Here's how the part is built. I have some questions about the finished solid (model axes, mm). A direction names the side the tool comes from. Give positions to 0.01 mm unless a question says otherwise; leave off trailing zeros. Order: outer loops, then holes, each group sorted by start corner. A loop starts at its lowest first (then second) coordinate and runs counter-clockwise, first axis right, second up.
from build123d import *

# Parameters (mm, degrees)
F0_R     = 10
F0_R_2   = 7.5
F1_DEPTH = 30
F2_R     = 4
F3_DEPTH = 2.5
F4_R     = 7.5
F5_DEPTH = 30.001


with BuildPart() as f1:
    # F0 (on Front) → F1 (new body)
    with BuildSketch(Plane.XZ):
        Circle(F0_R)
        Circle(F0_R_2, mode=Mode.SUBTRACT)
    extrude(amount=F1_DEPTH)

    # F2 (on Right) → F3 (join, symmetric)
    with BuildSketch(Plane.YZ):
        with BuildLine():
            Line((-22.5, 0.945997), (-7.5, 0.945997))
            Line((-7.5, 0.945997), (-7.5, 30.945997))
            ThreePointArc((-7.5, 30.945997), (-15, 38.445997), (-22.5, 30.945997))
            Line((-22.5, 30.945997), (-22.5, 0.945997))
        make_face()
        with Locations((-15, 30.945997)):
            Circle(F2_R, mode=Mode.SUBTRACT)
        with BuildLine():
            Line((-7.5, -29.054003), (-7.5, 0.945997))
            Line((-7.5, 0.945997), (-22.5, 0.945997))
            Line((-22.5, 0.945997), (-22.5, -29.054003))
            ThreePointArc((-22.5, -29.054003), (-15, -36.554003), (-7.5, -29.054003))
        make_face()
        with Locations((-15, -29.054003)):
            Circle(F2_R, mode=Mode.SUBTRACT)
    extrude(amount=F3_DEPTH, both=True)

    # F4 (on face) → F5 (cut, through all)
    with BuildSketch(Plane.XZ.offset(30)):
        Circle(F4_R)
    extrude(amount=-F5_DEPTH, mode=Mode.SUBTRACT)


solid = f1.part
Q1. If we section it at A-A on y = -15: List the corners of the cut face in (x, z) for me, plus the area to 3 significant figures.
Filled sheet:
outline: (-2.5, -36.55) - (2.5, -36.55) - (2.5, -33.05) - (-2.5, -33.05) - close; (-2.5, -25.05) - (2.5, -25.05) - (2.5, -9.68) arc R10 ccw to (2.5, 9.68) - (2.5, 26.95) - (-2.5, 26.95) - (-2.5, 9.68) arc R10 ccw to (-2.5, -9.68) - close; (-2.5, 34.95) - (2.5, 34.95) - (2.5, 38.45) - (-2.5, 38.45) - close; hole circle Ø15 at (0, 0)
area: 333 mm2
Q2. I need wall thicknesses on L1, parallel to Z at x = 0.5, y = -15; L2, parallel to X at y = -19, z = -12.5; L3, parallel to X at y = -28, z = 3. Which ranges of each line are inside material? Lowest first, please.
Filled sheet:
L1: z = -36.55 to -33.05, -25.05 to -7.48, 7.48 to 26.95, 34.95 to 38.45
L2: x = -2.5 to 2.5
L3: x = -9.54 to -6.87, 6.87 to 9.54
Q3. For faces 4 (the face through (-2.5, -15, 21)), 5 (the face through (4, -30, 7)), 6 (the face through (4, 0, 7)), 7 (the face through (-2.5, -15, -20)), 8 (the face through (2.5, -15, -20)), which set-ups out of +Z, -Z, +X, -X, +Y, -Y let a thin tool reach every point of the face, with its end or its side?
Filled sheet:
face 4: +Z, -X, +Y, -Y
face 5: +Z, -Z, +X, -X, -Y
face 6: +Z, -Z, +X, -X, +Y
face 7: -Z, -X, +Y, -Y
face 8: -Z, +X, +Y, -Y
Q4. I'm going to push flat-ended pins straight in: P1, Ø7.5, axis at y = -12.5, z = 30.5, coming from the -X side; P2, Ø5.5, axis at x = -1, z = 20.5, coming from the -Y side; P3, Ø4, axis at x = -0.5, z = -20.5, coming from the +Y side; P4, Ø6.5, axis at y = -15, z = 30.95, coming from the +X side. Where does each tip first touch, or does it pass through?
Filled sheet:
P1: stops at x = -2.5
P2: stops at y = -22.5
P3: stops at y = -7.5
P4: passes through
Q5. If we section it at D-D on x = -4.75: List the corners of the cut face in (y, z) for me, plus the area to 3 significant figures.
Filled sheet:
outline: (-30, -8.8) - (0, -8.8) - (0, -5.8) - (-30, -5.8) - close; (-30, 5.8) - (0, 5.8) - (0, 8.8) - (-30, 8.8) - close
area: 180 mm2
Q6. If we section it at C-C on x = -1.25: List the corners of the cut face in (y, z) for me.
Filled sheet:
outline: (-30, -9.92) - (-22.5, -9.92) - (-22.5, -29.05) arc R7.5 ccw to (-7.5, -29.05) - (-7.5, -9.92) - (0, -9.92) - (0, -7.4) - (-30, -7.4) - close; (-30, 7.4) - (0, 7.4) - (0, 9.92) - (-7.5, 9.92) - (-7.5, 30.95) arc R7.5 ccw to (-22.5, 30.95) - (-22.5, 9.92) - (-30, 9.92) - close; hole circle Ø8 at (-15, -29.05); hole circle Ø8 at (-15, 30.95)
Q7. If we section it at B-B on z = 0: List the corners of the cut face in (x, y) for me.
Filled sheet:
outline: (-10, -30) - (-7.5, -30) - (-7.5, 0) - (-10, 0) - close; (7.5, -30) - (10, -30) - (10, 0) - (7.5, 0) - close
Q8. Thinking about a two-plate mould opening in Y: for faces 1 (the face through (2.5, -15, 21)), 2 (the face through (0.035, -14.835, 38.444)), 3 (the face through (-0.035, -18.174, -31.488)), which applies, released by +Y, released by -Y, zero draft, split by the parting line, or undercut?
Filled sheet:
face 1: zero draft
face 2: split by the parting line
face 3: undercut
